from build123d import *

# Parameters (mm, degrees)
F0_W     = 10
F0_H     = 6
F1_DEPTH = 10
F2_R     = 2
F3_DEPTH = 6
F4_R     = 2


with BuildPart() as f1:
    # F0 (on Front) → F1 (new body)
    with BuildSketch(Plane.XZ):
        with Locations((-28.25, -20.25)):
            Rectangle(F0_W, F0_H)
        with Locations((28.25, -20.25)):
            Rectangle(F0_W, F0_H)
        with BuildLine():
            ThreePointArc((-17.25, 0), (0, 17.25), (17.25, 0))
            Line((17.25, 0), (17.25, -23.25))
            Line((17.25, -23.25), (23.25, -23.25))
            Line((23.25, -23.25), (23.25, -17.25))
            Line((23.25, -17.25), (23.25, 0))
            ThreePointArc((23.25, 0), (0, 23.25), (-23.25, 0))
            Line((-23.25, 0), (-23.25, -17.25))
            Line((-23.25, -17.25), (-23.25, -23.25))
            Line((-23.25, -23.25), (-17.25, -23.25))
            Line((-17.25, -23.25), (-17.25, 0))
        make_face()
    extrude(amount=F1_DEPTH)

    # F2 (on face) → F3 (cut, through all)
    with BuildSketch(Plane.XY.offset(-17.25)):
        with Locations((-28.25, -5)):
            Circle(F2_R)
        with Locations((28.25, -5)):
            Circle(F2_R)
    extrude(amount=-F3_DEPTH, mode=Mode.SUBTRACT)

    # F4
    f4_edges = [f1.edges().sort_by_distance(p)[0] for p in [
        (-23.25, -5, -17.25),
        (23.25, -5, -17.25),
        (33.25, -5, -17.25),
        (-33.25, -5, -17.25),
    ]]
    fillet(f4_edges, radius=F4_R)


solid = f1.part
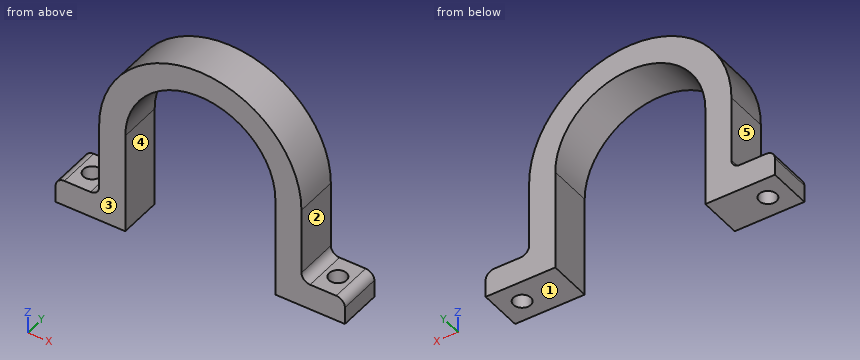
CAD build for the part. Positions are in the model's coordinates, mm. Face numbers are marked on the shaded views. A direction names the side the tool comes from. Round coordinates to 2 decimals unless told otherwise and drop trailing zeros. Loops run counter-clockwise (first coordinate to the right, second up) from the corner with the lowest first, then second, coordinate; pieces in that order, holes last.
(1) Which spindle directions (+Z, -Z, +X, -X, +Y, -Y) get a long thin tool onto all of the face, cutting with end or side? Do the marked faces 1, 2, 3, 4 and 5. Say none if no direction does.
(2) Wall check: line 1 along X through (y, z) = (-0.75, -8.5); line 2 along Y through (x, z) = (28.25, -19.45); line 3 along X through (y, z) = (-8.75, -15.5). Give the ranges that are in metal, low to high.
(3) Drop flat-ended pins along their axis: pin 1 (5 mm diameter, centred on x = -9, z = 11, fed in from -Y); pin 2 (5 mm diameter, centred on x = -28, y = -4.5, fed in from +Z); pin 3 (6 mm diameter, centred on x = 7.5, z = 16.5, fed in from +Y); pin 4 (5 mm diameter, centred on y = -7, z = -14, fed in from -X). Give the stop position or say it passes through.
(4) Cut at A-A (y = -5). Give the cut face in (x, z).
(5) Cut at D-D (y = -8). Give the cut face in (x, z).
(6) Cut at C-C (z = -14.5). Give the cut face in (x, y), plus the area to 3 significant figures.
(7) Cut at B-B (x = -28.25). Give the cut face in (y, z), plus the area to 3 significant figures.
Findings below:
1. face 1: -Z, +X, -X, +Y, -Y
1. face 2: +Z, +X, +Y, -Y
1. face 3: +Z, -Z, +X, -X, -Y
1. face 4: -Z, +Y, -Y
1. face 5: +Z, -X, +Y, -Y
2. line 1: x = -23.25 to -17.25, 17.25 to 23.25
2. line 2: y = -10 to -7, -3 to 0
2. line 3: x = -23.27 to -17.25, 17.25 to 23.27
3. pin 1: passes through
3. pin 2: stops at z = -17.25
3. pin 3: stops at y = 0
3. pin 4: stops at x = -23.69
4. outline: (-33.25, -23.25) - (-30.25, -23.25) - (-30.25, -17.25) - (-31.25, -17.25) arc R2 ccw to (-33.25, -19.25) - close; (-26.25, -23.25) - (-17.25, -23.25) - (-17.25, 0) arc R17.25 cw to (17.25, 0) - (17.25, -23.25) - (26.25, -23.25) - (26.25, -17.25) - (25.25, -17.25) arc R2 cw to (23.25, -15.25) - (23.25, 0) arc R23.25 ccw to (-23.25, 0) - (-23.25, -15.25) arc R2 cw to (-25.25, -17.25) - (-26.25, -17.25) - close; (30.25, -23.25) - (33.25, -23.25) - (33.25, -19.25) arc R2 ccw to (31.25, -17.25) - (30.25, -17.25) - close
5. outline: (-33.25, -23.25) - (-17.25, -23.25) - (-17.25, 0) arc R17.25 cw to (17.25, 0) - (17.25, -23.25) - (33.25, -23.25) - (33.25, -19.25) arc R2 ccw to (31.25, -17.25) - (25.25, -17.25) arc R2 cw to (23.25, -15.25) - (23.25, 0) arc R23.25 ccw to (-23.25, 0) - (-23.25, -15.25) arc R2 cw to (-25.25, -17.25) - (-31.25, -17.25) arc R2 ccw to (-33.25, -19.25) - close
6. outline: (-23.25, -10) - (-17.25, -10) - (-17.25, 0) - (-23.25, 0) - close; (17.25, -10) - (23.25, -10) - (23.25, 0) - (17.25, 0) - close
6. area: 120 mm2
7. outline: (-10, -23.25) - (-7, -23.25) - (-7, -17.25) - (-10, -17.25) - close; (-3, -23.25) - (0, -23.25) - (0, -17.25) - (-3, -17.25) - close
7. area: 36.0 mm2
